Check sheet for the modelled part. Datum: model origin and axes. Units: mm. Coordinates: 2 decimals unless noted, no trailing zeros. Loops run counter-clockwise (first coordinate to the right, second up) from the corner with the lowest first, then second, coordinate; pieces in that order, holes last.
```python
from build123d import *

# Parameters (mm, degrees)
CYLINDER007_R     = 2
CYLINDER007_DEPTH = 25
CYLINDER008_R     = 2
CYLINDER008_DEPTH = 25
CYLINDER006_R     = 2
CYLINDER006_DEPTH = 25
CYLINDER009_R     = 2
CYLINDER009_DEPTH = 25
CYLINDER005_R     = 2
CYLINDER005_DEPTH = 25
CYLINDER002_R     = 2
CYLINDER002_DEPTH = 25
CYLINDER001_R     = 2
CYLINDER001_DEPTH = 25
CYLINDER_R        = 2
CYLINDER_DEPTH    = 25
CYLINDER003_R     = 2
CYLINDER003_DEPTH = 25
CYLINDER004_R     = 2
CYLINDER004_DEPTH = 25
BOX_W             = 50
BOX_H             = 130
BOX_DEPTH         = 18


with BuildPart() as cilindro007:
    # Cylinder007 → Cylinder007 (new body)
    with BuildSketch(Plane(origin=(6, 76, 0), x_dir=(1, 0, 0), z_dir=(0, 0, 1))):
        Circle(CYLINDER007_R)
    extrude(amount=CYLINDER007_DEPTH)


with BuildPart() as cilindro008:
    # Cylinder008 → Cylinder008 (new body)
    with BuildSketch(Plane(origin=(30, 58, 0), x_dir=(1, 0, 0), z_dir=(0, 0, 1))):
        Circle(CYLINDER008_R)
    extrude(amount=CYLINDER008_DEPTH)


with BuildPart() as cilindro006:
    # Cylinder006 → Cylinder006 (new body)
    with BuildSketch(Plane(origin=(6, 58, 0), x_dir=(1, 0, 0), z_dir=(0, 0, 1))):
        Circle(CYLINDER006_R)
    extrude(amount=CYLINDER006_DEPTH)


with BuildPart() as huecos001:
    # Cylinder009 → Cylinder009 (new body)
    with BuildSketch(Plane(origin=(30, 76, 0), x_dir=(1, 0, 0), z_dir=(0, 0, 1))):
        Circle(CYLINDER009_R)
    extrude(amount=CYLINDER009_DEPTH)

    # Fusion001: union Cilindro007, Cilindro008, Cilindro006
    add(cilindro007.part)
    add(cilindro008.part)
    add(cilindro006.part)


with BuildPart() as huecos001_1:
    # Fusion001 placement: moved
    add(huecos001.part.moved(Location((0, 49, 0))))


with BuildPart() as cilindro005:
    # Cylinder005 → Cylinder005 (new body)
    with BuildSketch(Plane(origin=(31, 91.5, 0), x_dir=(1, 0, 0), z_dir=(0, 0, 1))):
        Circle(CYLINDER005_R)
    extrude(amount=CYLINDER005_DEPTH)


with BuildPart() as cilindro002:
    # Cylinder002 → Cylinder002 (new body)
    with BuildSketch(Plane(origin=(6, 76, 0), x_dir=(1, 0, 0), z_dir=(0, 0, 1))):
        Circle(CYLINDER002_R)
    extrude(amount=CYLINDER002_DEPTH)


with BuildPart() as cilindro001:
    # Cylinder001 → Cylinder001 (new body)
    with BuildSketch(Plane(origin=(30, 58, 0), x_dir=(1, 0, 0), z_dir=(0, 0, 1))):
        Circle(CYLINDER001_R)
    extrude(amount=CYLINDER001_DEPTH)


with BuildPart() as cilindro:
    # Cylinder → Cylinder (new body)
    with BuildSketch(Plane(origin=(6, 58, 0), x_dir=(1, 0, 0), z_dir=(0, 0, 1))):
        Circle(CYLINDER_R)
    extrude(amount=CYLINDER_DEPTH)


with BuildPart() as huecos:
    # Cylinder003 → Cylinder003 (new body)
    with BuildSketch(Plane(origin=(30, 76, 0), x_dir=(1, 0, 0), z_dir=(0, 0, 1))):
        Circle(CYLINDER003_R)
    extrude(amount=CYLINDER003_DEPTH)

    # Fusion: union Cilindro002, Cilindro001, Cilindro
    add(cilindro002.part)
    add(cilindro001.part)
    add(cilindro.part)


with BuildPart() as cilindro004:
    # Cylinder004 → Cylinder004 (new body)
    with BuildSketch(Plane(origin=(11, 32.5, 0), x_dir=(1, 0, 0), z_dir=(0, 0, 1))):
        Circle(CYLINDER004_R)
    extrude(amount=CYLINDER004_DEPTH)


with BuildPart() as izquierda:
    # Box → Box (new body)
    with BuildSketch(Plane.XY):
        with Locations((25, 65)):
            Rectangle(BOX_W, BOX_H)
    extrude(amount=BOX_DEPTH)

    # Cut: cut Cilindro004
    add(cilindro004.part, mode=Mode.SUBTRACT)

    # Cut001: cut Huecos
    add(huecos.part, mode=Mode.SUBTRACT)

    # Cut002: cut Cilindro005
    add(cilindro005.part, mode=Mode.SUBTRACT)

    # Cut003: cut Huecos001
    add(huecos001_1.part, mode=Mode.SUBTRACT)


with BuildPart() as fusion002:
    # mirror: instance of Izquierda
    add(izquierda.part.mirror(Plane(origin=(50, 0, 0.197234), x_dir=(0, -1, 0), z_dir=(1, 0, 0))))

    # Fusion002: union Izquierda
    add(izquierda.part)


solid = fusion002.part
```
1) Section check B-B on z = 10. Give the number of separate pieces and of enclosed holes in the cut face, plus the area to 3 significant figures.
Answer sheet:
separate pieces: 1
enclosed holes: 20
area: 12,700 mm2
2) Section check C-C on y = 107. Enter the section's corners in (x, z).
Answer sheet:
outline: (0, 0) - (4, 0) - (4, 18) - (0, 18) - close; (8, 0) - (28, 0) - (28, 18) - (8, 18) - close; (32, 0) - (68, 0) - (68, 18) - (32, 18) - close; (72, 0) - (92, 0) - (92, 18) - (72, 18) - close; (96, 0) - (100, 0) - (100, 18) - (96, 18) - close
3) Scan lines: line 1 (X direction, y = 125, z = 11.5); line 2 (Y direction, x = 94, z = 6.5); line 3 (Y direction, x = 4.5, z = 5). Record each from-to range of solid material in increasing order.
Answer sheet:
line 1: x = 0 to 4, 8 to 28, 32 to 68, 72 to 92, 96 to 100
line 2: y = 0 to 56, 60 to 74, 78 to 105, 109 to 123, 127 to 130
line 3: y = 0 to 56.68, 59.32 to 74.68, 77.32 to 105.68, 108.32 to 123.68, 126.32 to 130
4) Section check D-D on y = 91.5. Enter the section's corners in (x, z), plus the area to 3 significant figures.
Answer sheet:
outline: (0, 0) - (29, 0) - (29, 18) - (0, 18) - close; (33, 0) - (67, 0) - (67, 18) - (33, 18) - close; (71, 0) - (100, 0) - (100, 18) - (71, 18) - close
area: 1,660 mm2
5) Mould release check, pull along Y, two halves, no side actions. Record for faces 1 (the cylindrical face through (92.092, 58.601, 8.874)), 2 (the flat face through (49, 66, 0)), 3 (the flat face through (49, 0, 9)): +Y half, -Y half, draft (parallel to the pull), parting line (faces both ways), or undercut.
Answer sheet:
face 1: undercut
face 2: draft
face 3: -Y half
6) Section check A-A on x = 94. Enter the section's corners in (y, z), plus the area to 3 significant figures.
Answer sheet:
outline: (0, 0) - (56, 0) - (56, 18) - (0, 18) - close; (60, 0) - (74, 0) - (74, 18) - (60, 18) - close; (78, 0) - (105, 0) - (105, 18) - (78, 18) - close; (109, 0) - (123, 0) - (123, 18) - (109, 18) - close; (127, 0) - (130, 0) - (130, 18) - (127, 18) - close
area: 2,050 mm2
